from build123d import *

# Parameters (mm, degrees)
CYLINDER019_R     = 1
CYLINDER019_DEPTH = 40
CYLINDER018_R     = 1
CYLINDER018_DEPTH = 40
BOX011_W          = 22
BOX011_H          = 22
BOX011_DEPTH      = 20
FILLET004_R       = 2
CYLINDER017_R     = 16
CYLINDER017_DEPTH = 4
FILLET003_R       = 1


with BuildPart() as screw_hole_cylinder003:
    # Cylinder019 → Cylinder019 (new body)
    with BuildSketch(Plane(origin=(0, 20, 7), x_dir=(0, 0, -1), z_dir=(0, -1, 0))):
        Circle(CYLINDER019_R)
    extrude(amount=CYLINDER019_DEPTH)


with BuildPart() as obj1:
    # Cylinder018 → Cylinder018 (new body)
    with BuildSketch(Plane(origin=(-20, 0, 15), x_dir=(0, 0, -1), z_dir=(1, 0, 0))):
        Circle(CYLINDER018_R)
    extrude(amount=CYLINDER018_DEPTH)

    # Fusion018: union screw hole cylinder003
    add(screw_hole_cylinder003.part)


with BuildPart() as fillet004:
    # Box011 → Box011 (new body)
    with BuildSketch(Plane(origin=(-11, -11, 0), x_dir=(1, 0, 0), z_dir=(0, 0, 1))):
        with Locations((11, 11)):
            Rectangle(BOX011_W, BOX011_H)
    extrude(amount=BOX011_DEPTH)

    # Fillet004
    fillet004_edges = [fillet004.edges().sort_by_distance(p)[0] for p in [
        (-11, -11, 10),
        (-11, 11, 10),
        (11, -11, 10),
        (11, 11, 10),
    ]]
    fillet(fillet004_edges, radius=FILLET004_R)


with BuildPart() as top_cut:
    # Cylinder017 → Cylinder017 (new body)
    with BuildSketch(Plane.XY.offset(20)):
        Circle(CYLINDER017_R)
    extrude(amount=CYLINDER017_DEPTH)

    # Fillet003
    fillet003_edges = [top_cut.edges().sort_by_distance(p)[0] for p in [
        (-16, 0, 24),
        (-16, 0, 20),
    ]]
    fillet(fillet003_edges, radius=FILLET003_R)

    # Fusion017: union Fillet004
    add(fillet004.part)

    # Cut005: cut obj1
    add(obj1.part, mode=Mode.SUBTRACT)


solid = top_cut.part
Verification items for the finished model (mm, model axes). A direction names the side the tool comes from. Give positions to 0.01 mm unless a question says otherwise; leave off trailing zeros. Loops run counter-clockwise (first coordinate to the right, second up) from the corner with the lowest first, then second, coordinate; pieces in that order, holes last. Notation, with made-up numbers: (15, 41) - (44, 41) arc R11 cw to (44, 59) - close; hole circle Ø4 at (-38.5, 77). An arc over 180 degrees is marked (long way). Write each question's results on one line, items separated by ' | '.
1) Mould release check, pull along X, two halves, no side actions. Record for faces 6 (the cylindrical face through (-0.6, 0.2, 7.8)), 7 (the cylindrical face through (10.4, -10.43, 10.14)), 8 (the flat face through (0, 0, 0)), 9 (the cylindrical face through (-3.47, -15.62, 21.99)): pulls with the +X half, pulls with the -X half, needs draft (parallel to the pull), parting line crosses it, or undercut.
Solution:
face 6: undercut | face 7: pulls with the +X half | face 8: needs draft | face 9: parting line crosses it
2) Sectioned sample at B-B on z = 7. Record the boundary of the cut face in (x, y).
Solution:
outline: (-11, -9) arc R2 ccw to (-9, -11) - (-1, -11) - (-1, 11) - (-9, 11) arc R2 ccw to (-11, 9) - close; (1, -11) - (9, -11) arc R2 ccw to (11, -9) - (11, 9) arc R2 ccw to (9, 11) - (1, 11) - close
3) Sectioned sample at C-C on x = 0. Record the boundary of the cut face in (y, z).
Solution:
outline: (-16, 21) arc R1 ccw to (-15, 20) - (-11, 20) - (-11, 8) - (11, 8) - (11, 20) - (15, 20) arc R1 ccw to (16, 21) - (16, 23) arc R1 ccw to (15, 24) - (-15, 24) arc R1 ccw to (-16, 23) - close; (-11, 0) - (11, 0) - (11, 6) - (-11, 6) - close; hole circle Ø2 at (0, 15)
4) Depth check by flat-ended pin: P1, Ø4, axis at y = 3.5, z = 9, coming from the +X side; P2, Ø10, axis at x = -9, z = 14, coming from the -Y side; P3, Ø1.6, axis at y = 0, z = 15, coming from the -X side. Enter the tip coordinate at first touch or a pass-through.
Solution:
P1: x = 11 | P2: y = -11 | P3: through
5) Sectioned sample at D-D on z = 12.25. Record the boundary of the cut face in (x, y).
Solution:
outline: (-11, -9) arc R2 ccw to (-9, -11) - (9, -11) arc R2 ccw to (11, -9) - (11, 9) arc R2 ccw to (9, 11) - (-9, 11) arc R2 ccw to (-11, 9) - close
6) Material ranges on L1, parallel to Y at x = -6.25, z = 15; L2, parallel to Z at x = 0, y = 2; L3, parallel to Z at x = -5, y = 0, recorded low to high. Write a range as from..to.
Solution:
L1: -11..-1, 1..11 | L2: 0..6, 8..24 | L3: 0..14, 16..24
7) Tool access check on faces 1 (the flat face through (0, 11, 10)), 2 (the cylindrical face through (-10.43, 10.4, 10.14)), 3 (the cylindrical face through (-10.43, -10.4, 10.14)), 4 (the flat face through (0, -11, 10)), 5 (the flat face through (-11, 0, 10)). Record the directions out of +Z, -Z, +X, -X, +Y, -Y that give a thin tool (end or side, any length) a straight path to the whole face; none if there is none.
Solution:
face 1: -Z, +X, -X, +Y | face 2: -Z, -X, +Y | face 3: -Z, -X, -Y | face 4: -Z, +X, -X, -Y | face 5: -Z, -X, +Y, -Y
8) Sectioned sample at A-A on y = 0. Record the boundary of the cut face in (x, z).
Solution:
outline: (-16, 21) arc R1 ccw to (-15, 20) - (-11, 20) - (-11, 16) - (11, 16) - (11, 20) - (15, 20) arc R1 ccw to (16, 21) - (16, 23) arc R1 ccw to (15, 24) - (-15, 24) arc R1 ccw to (-16, 23) - close; (-11, 0) - (11, 0) - (11, 14) - (-11, 14) - close; hole circle Ø2 at (0, 7)
